Geometry: final body of the model. Coordinates: model frame, mm. Give positions to 0.01 mm unless a question says otherwise; leave off trailing zeros. Write each loop counter-clockwise with the first axis right and the second up, starting at its lowest first coordinate (ties: lowest second). Pieces come first, ordered by that corner, then holes. Notation, with made-up numbers: (26, 73) - (49, 73) arc R19 cw to (49, 109) - close; hole circle Ø4 at (-38.5, 50.5). An arc over 180 degrees is marked (long way). Use CSV: the item, a comma, the result in double quotes. Start each with the question number.
(1) Section C-C on z = 143.5. Output: boundary loops of the cut face in (x, y) (3 decimals).
(2) Section D-D on z = 110.5. Output: boundary loops of the cut face in (x, y) (3 decimals), and give its area (3 significant figures).
(3) Section A-A on x = 8.5. Output: boundary loops of the cut face in (y, z) (3 decimals).
(4) Line query: probe 1 along X at (y, z) = (6.5, 57) (3 decimals); probe 2 along X at (y, z) = (0, 13.5). Output: solid intervals per line, ascending. Write a range as [from, to].
(5) First-contact query: pin 1 Ø7 at (x, z) = (-1, 70.5) entering from +Y; pin 2 Ø3 at (x, z) = (1.5, 81.5) entering from -Y; pin 3 Ø5 at (y, z) = (-0.5, 97.5) entering from +X; pin 4 Ø1.9 at (y, z) = (-0.5, 87.5) entering from -X. Flat tips, straight axial feed; report the tip coordinate or a pass-through.
from build123d import *

# Parameters (mm, degrees)
BOSS_EXTRU_1_DEPTH = 160


with BuildPart() as part:
    # Esquisse1 → Boss.-Extru.1 (new body)
    with BuildSketch(Plane.XY):
        Polygon((3.125, 11), (11, 11), (11, 3.125), (5, 3.125), (5, -3.125), (11, -3.125), (11, -11), (3.125, -11), (3.125, -5), (-3.125, -5), (-3.125, -11), (-11, -11), (-11, -3.125), (-5, -3.125), (-5, 3.125), (-11, 3.125), (-11, 11), (-3.125, 11), (-3.125, 5), (3.125, 5), align=None)
    extrude(amount=BOSS_EXTRU_1_DEPTH)

    # Esquisse3 → Dégagement M61 (revolve, cut)
    with BuildSketch(Plane(origin=(0, 0, 160), x_dir=(0, -1, 0), z_dir=(1, 0, 0))):
        Polygon((0, 0), (0, 25), (3.3, 23.017159957), (3.3, 0), align=None)
    d_gagement_m61 = revolve(axis=Axis((0, 0, 166.35), (0, 0, -1)), mode=Mode.SUBTRACT)

    # Symétrie1: Dégagement M61 across plane
    add(d_gagement_m61.mirror(Plane.XY.offset(80)), mode=Mode.SUBTRACT)


solid = part.part
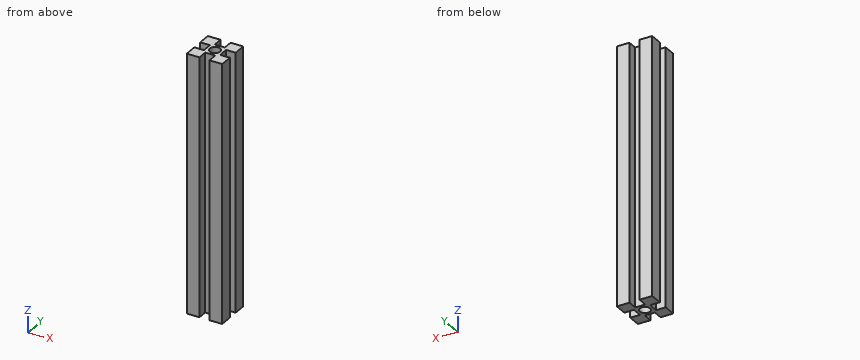
Check values:
1,outline,"(-11, -11) - (-3.125, -11) - (-3.125, -5) - (3.125, -5) - (3.125, -11) - (11, -11) - (11, -3.125) - (5, -3.125) - (5, 3.125) - (11, 3.125) - (11, 11) - (3.125, 11) - (3.125, 5) - (-3.125, 5) - (-3.125, 11) - (-11, 11) - (-11, 3.125) - (-5, 3.125) - (-5, -3.125) - (-11, -3.125) - close; hole circle Ø6.6 at (0, 0)"
2,outline,"(-11, -11) - (-3.125, -11) - (-3.125, -5) - (3.125, -5) - (3.125, -11) - (11, -11) - (11, -3.125) - (5, -3.125) - (5, 3.125) - (11, 3.125) - (11, 11) - (3.125, 11) - (3.125, 5) - (-3.125, 5) - (-3.125, 11) - (-11, 11) - (-11, 3.125) - (-5, 3.125) - (-5, -3.125) - (-11, -3.125) - close"
2,area,"334 mm²"
3,outline,"(-11, 0) - (-3.125, 0) - (-3.125, 160) - (-11, 160) - close; (3.125, 0) - (11, 0) - (11, 160) - (3.125, 160) - close"
4,probe 1,"x = [-11, -3.125], [3.125, 11]"
4,probe 2,"x = [-5, -3.3], [3.3, 5]"
5,pin 1,"stops at y = 11"
5,pin 2,"stops at y = -5"
5,pin 3,"stops at x = 5"
5,pin 4,"stops at x = -5"
